Input: part model. Units: mm. Frame: model coordinates. Coordinates: 2 decimals unless noted, no trailing zeros. Write each loop counter-clockwise with the first axis right and the second up, starting at its lowest first coordinate (ties: lowest second). Pieces come first, ordered by that corner, then holes. Notation, with made-up numbers: M 72,5.5 L 126,5.5 A11 ccw 126,23.5 Z; hole C 46,64.25 d11. An arc over 180 degrees is marked long. Use one line per item in the form item = value.
from build123d import *

# Parameters (mm, degrees)
BOSS_EXTRUDE1_DEPTH      = 2.5
BOSS_EXTRUDE2_DEPTH      = 8.5
BOSS_EXTRUDE2_DEPTH_BACK = 3.25
SKETCH2_W                = 0.75
SKETCH2_H                = 0.75
CHAMFER1_SIZE            = 0.3


with BuildPart() as part:
    # Sketch1 → Boss-Extrude1 (new body)
    with BuildSketch(Plane(origin=(0, 0, 0), x_dir=(-1, 0, 0), z_dir=(0, 1, 0))):
        with BuildLine():
            Line((-22.25, 1.27), (2, 1.27))
            ThreePointArc((2, 1.27), (2.353553391, 1.123553391), (2.5, 0.77))
            Line((2.5, 0.77), (2.5, -0.77))
            ThreePointArc((2.5, -0.77), (2.353553391, -1.123553391), (2, -1.27))
            Line((2, -1.27), (-22.25, -1.27))
            ThreePointArc((-22.25, -1.27), (-22.603553391, -1.123553391), (-22.75, -0.77))
            Line((-22.75, -0.77), (-22.75, 0.77))
            ThreePointArc((-22.75, 0.77), (-22.603553391, 1.123553391), (-22.25, 1.27))
        make_face()
    extrude(amount=BOSS_EXTRUDE1_DEPTH)

    # Sketch2 → Boss-Extrude2 (add, two sides: drawn at the far end of the back side and taken through both)
    with BuildSketch(Plane(origin=(0, 0, 0), x_dir=(-1, 0, 0), z_dir=(0, 1, 0)).offset(-BOSS_EXTRUDE2_DEPTH_BACK)):
        with Locations((1.27, 0)):
            Rectangle(SKETCH2_W, SKETCH2_H)
        with Locations((-1.27, 0)):
            Rectangle(SKETCH2_W, SKETCH2_H)
        with Locations((-3.81, 0)):
            Rectangle(SKETCH2_W, SKETCH2_H)
        with Locations((-6.35, 0)):
            Rectangle(SKETCH2_W, SKETCH2_H)
        with Locations((-8.89, 0)):
            Rectangle(SKETCH2_W, SKETCH2_H)
        with Locations((-11.43, 0)):
            Rectangle(SKETCH2_W, SKETCH2_H)
        with Locations((-13.97, 0)):
            Rectangle(SKETCH2_W, SKETCH2_H)
        with Locations((-16.51, 0)):
            Rectangle(SKETCH2_W, SKETCH2_H)
        with Locations((-19.05, 0)):
            Rectangle(SKETCH2_W, SKETCH2_H)
        with Locations((-21.59, 0)):
            Rectangle(SKETCH2_W, SKETCH2_H)
    extrude(amount=BOSS_EXTRUDE2_DEPTH + BOSS_EXTRUDE2_DEPTH_BACK)

    # Chamfer1
    chamfer1_edges = [part.edges().sort_by_distance(p)[0] for p in [
        (9.265, -3.25, 0),
        (8.89, -3.25, 0.375),
        (8.515, -3.25, 0),
        (8.89, -3.25, -0.375),
        (9.265, 8.5, 0),
        (8.89, 8.5, -0.375),
        (8.515, 8.5, 0),
        (8.89, 8.5, 0.375),
        (11.055, -3.25, 0),
        (11.43, -3.25, -0.375),
        (11.805, -3.25, 0),
        (11.43, -3.25, 0.375),
        (11.055, 8.5, 0),
        (11.43, 8.5, 0.375),
        (11.805, 8.5, 0),
        (11.43, 8.5, -0.375),
        (14.345, -3.25, 0),
        (13.97, -3.25, 0.375),
        (13.595, -3.25, 0),
        (13.97, -3.25, -0.375),
        (14.345, 8.5, 0),
        (13.97, 8.5, -0.375),
        (13.595, 8.5, 0),
        (13.97, 8.5, 0.375),
        (16.135, -3.25, 0),
        (16.51, -3.25, -0.375),
        (16.885, -3.25, 0),
        (16.51, -3.25, 0.375),
        (16.135, 8.5, 0),
        (16.51, 8.5, 0.375),
        (16.885, 8.5, 0),
        (16.51, 8.5, -0.375),
        (19.425, -3.25, 0),
        (19.05, -3.25, 0.375),
        (18.675, -3.25, 0),
        (19.05, -3.25, -0.375),
        (19.425, 8.5, 0),
        (19.05, 8.5, -0.375),
        (18.675, 8.5, 0),
        (19.05, 8.5, 0.375),
        (21.215, -3.25, 0),
        (21.59, -3.25, -0.375),
        (21.965, -3.25, 0),
        (21.59, -3.25, 0.375),
        (21.215, 8.5, 0),
        (21.59, 8.5, 0.375),
        (21.965, 8.5, 0),
        (21.59, 8.5, -0.375),
        (-0.895, -3.25, 0),
        (-1.27, -3.25, 0.375),
        (-1.645, -3.25, 0),
        (-1.27, -3.25, -0.375),
        (-0.895, 8.5, 0),
        (-1.27, 8.5, -0.375),
        (-1.645, 8.5, 0),
        (-1.27, 8.5, 0.375),
        (0.895, -3.25, 0),
        (1.27, -3.25, -0.375),
        (1.645, -3.25, 0),
        (1.27, -3.25, 0.375),
        (0.895, 8.5, 0),
        (1.27, 8.5, 0.375),
        (1.645, 8.5, 0),
        (1.27, 8.5, -0.375),
        (4.185, -3.25, 0),
        (3.81, -3.25, 0.375),
        (3.435, -3.25, 0),
        (3.81, -3.25, -0.375),
        (4.185, 8.5, 0),
        (3.81, 8.5, -0.375),
        (3.435, 8.5, 0),
        (3.81, 8.5, 0.375),
        (5.975, -3.25, 0),
        (6.35, -3.25, -0.375),
        (6.725, -3.25, 0),
        (6.35, -3.25, 0.375),
        (5.975, 8.5, 0),
        (6.35, 8.5, 0.375),
        (6.725, 8.5, 0),
        (6.35, 8.5, -0.375),
    ]]
    chamfer(chamfer1_edges, length=CHAMFER1_SIZE)


solid = part.part
(1) Line query: probe 1 along Z at (x, y) = (-1, -0.5) (3 decimals); probe 2 along Y at (x, z) = (0.75, 0.45); probe 3 along Y at (x, z) = (3.5, 0.15) (3 decimals). Output: solid intervals per line, ascending.
Computed:
probe_1 = -0.375 to 0.375
probe_2 = 0 to 2.5
probe_3 = -3.015 to 8.265
(2) Section query A-A on y = -1.5. State how many separate pieces and enclosed holes the cut face has, plus the area to 4 significant figures.
Computed:
separate_pieces = 10
enclosed_holes = 0
area = 5.625 mm^2
(3) First-contact query: pin 1 Ø0.6 at (x, y) = (21.5, -1) entering from +Z (3 decimals); pin 2 Ø0.8 at (y, z) = (4, 0) entering from +X (3 decimals); pin 3 Ø0.6 at (x, y) = (9, 4.5) entering from -Z (3 decimals). Flat tips, straight axial feed; report the tip coordinate or a pass-through.
Computed:
pin_1 = 0.375
pin_2 = 21.965
pin_3 = -0.375
(4) Section query B-B on x = 3. Return the cut outline in (y, z), plus the area to 3 significant figures.
Computed:
outline = M 0,-1.27 L 2.5,-1.27 L 2.5,1.27 L 0,1.27 Z
area = 6.35 mm^2
